Autodesk Inventor part; units mm, degrees
ref_plane "YZ Plane" through (0, 0, 0) normal (1, 0, 0) x (0, 1, 0)
ref_plane "XZ Plane" through (0, 0, 0) normal (0, 1, 0) x (-1, 0, 0)
ref_plane "XY Plane" through (0, 0, 0) normal (0, 0, 1) x (1, 0, 0)
sketch "Sketch1" plane through (0, 0, 0) normal (1, 0, 0) x (0, 1, 0)
  line L0 (0, 0) -> (47.0027, 0)
  line L1 (47.0027, 0) -> (47.0027, -9.525)
  line L2 (47.0027, -9.525) -> (0, -9.525)
  line L3 (0, -9.525) -> (0, 0)
  dimension "d0" = 47.0027
  dimension "d1" = 9.525
revolve "Revolution1" add sketch "Sketch1" angle 360 about axis through (0, 0, -9.525) along (0, 0, 1)
sketch "Sketch2" plane through (0, 0, 0) normal (0, 0, 1) x (1, 0, 0)
  circle A0 centre (0, 0) radius 39.0906
  line L0 (0, 0) -> (27.6412, 27.6412)
  line L1 (0, 0) -> (39.0906, 0) construction
  circle A1 centre (27.6412, 27.6412) radius 3.4036
  circle A2 centre (37.7586, -10.1174) radius 3.4036
  circle A3 centre (10.1174, -37.7586) radius 3.4036
  circle A4 centre (-27.6412, -27.6412) radius 3.4036
  circle A5 centre (-37.7586, 10.1174) radius 3.4036
  circle A6 centre (-10.1174, 37.7586) radius 3.4036
  point P0 (0, 0)
  dimension "d3" = 78.1812
  dimension "d4" = 45
  dimension "d5" = 6.8072
  dimension "d8" = 360
extrude "Extrusion1" cut sketch "Sketch2" against normal blind 9.525 contours A1 L0 A0 | A0 A1 | A2 A0 | A0 A2 | L0 A1 A0 | A3 A0 | A0 A3 | A6 A0 | A0 A6 | A4 A0 | A0 A4 | A5 A0 | A0 A5
sketch "Sketch3" plane through (0, 0, 0) normal (0, 0, 1) x (1, 0, 0)
  circle A0 centre (0, 0) radius 31.1277
  line L0 (0, 0) -> (-22.0106, 22.0106)
  line L1 (0, 0) -> (31.1277, 0) construction
  circle A1 centre (-27.6412, -27.6412) radius 3.4036
  circle A2 centre (-22.0106, 22.0106) radius 5.08
  circle A3 centre (-8.0564, -30.067) radius 5.08
  circle A4 centre (30.067, 8.0564) radius 5.08
  circle A5 centre (0, 0) radius 15.875
  point P0 (0, 0)
  dimension "d12" = 62.2554
  dimension "d13" = 135
  dimension "d14" = 10.16
  dimension "d17" = 360
  dimension "d21" = 31.75
extrude "Extrusion2" cut sketch "Sketch3" against normal blind 9.525 contours A5 | A4 A0 | A0 A4 | A3 A0 | A0 A3 | A2 L0 A0 | A0 A2 | A0 L0 A2
chamfer "Chamfer1" distance 0.762 angle 45 12 edges at (-15.875, 0, 0) (0, -47.0027, 0) (0, -47.0027, -9.525) (24.987, 8.0564, 0) (24.2376, 27.6412, 0) (-13.521, 37.7586, 0) (-27.0906, 22.0106, 0) (-41.1622, 10.1174, 0) (-31.0448, -27.6412, 0) (-13.1364, -30.067, 0) (6.7138, -37.7586, 0) (34.355, -10.1174, 0)
properties part number "Motor_Adapter_Flex"
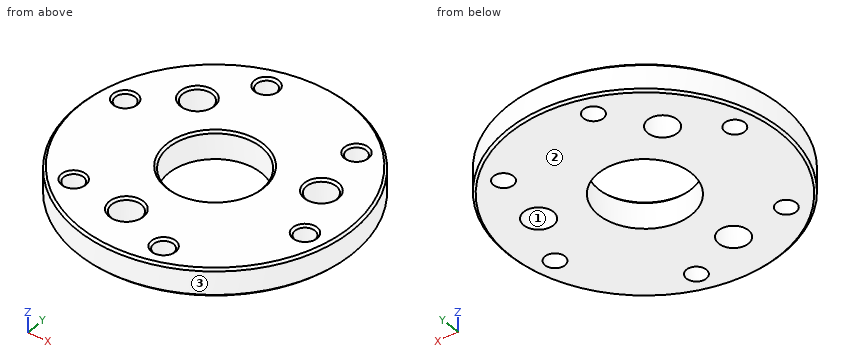
Could you check a few things on this model? Use its own coordinates, in mm. Face numbers are marked on the shaded views. Give positions to 0.01 mm unless a question says otherwise; leave off trailing zeros. Write each loop counter-clockwise with the first axis right and the second up, starting at its lowest first coordinate (ties: lowest second). Pieces come first, ordered by that corner, then holes. Notation, with made-up numbers: (37, -32) -> (81, -32) arc R29 cw to (81, -3) -> close; hole circle Ø9 at (15, 78.5). An arc over 180 degrees is marked (long way). Answer as a JSON object with one key per item and string values.
Q1. Suppose I cut it at A-A on x = 0. Write out the boundary of the cut face in (y, z) (3 decimals), then the cut area to 3 significant figures.
Taken from the geometry:
{"outline": "(-47.003, -8.763) -> (-46.241, -9.525) -> (-15.875, -9.525) -> (-15.875, -0.762) -> (-16.637, 0) -> (-46.241, 0) -> (-47.003, -0.762) -> close; (15.875, -9.525) -> (46.241, -9.525) -> (47.003, -8.763) -> (47.003, -0.762) -> (46.241, 0) -> (16.637, 0) -> (15.875, -0.762) -> close", "area": "591 mm²"}
Q2. We'd pull the mould along X, two halves only. Please class the marked faces 1, 2 and 3: released by +X, released by -X, zero draft, split by the parting line, or undercut.
Taken from the geometry:
{"face 1": "undercut", "face 2": "zero draft", "face 3": "split by the parting line"}
Q3. Please list where these lines run through material, in increasing order: L1, parallel to X at y = 0, z = -5.25 (3 decimals); L2, parallel to X at y = 26.5, z = -0.5; L3, parallel to Y at x = -3.5, z = -0.75.
Taken from the geometry:
{"L1": "x = -47.003 to -15.875, 15.875 to 47.003", "L2": "x = -38.5 to -24.91, -19.12 to 24.16, 31.12 to 38.5", "L3": "y = -46.86 to -32.34, -27.79 to -15.5, 15.5 to 46.86"}
Q4. Will these pins go through, and if not, where does the flat tip stop? pin 1 Ø3 at (x, z) = (-21, -4) entering from +Y; pin 2 Ø2 at (x, z) = (25, -8.5) entering from +Y; pin 3 Ø2 at (y, z) = (-25.5, -8) entering from -X.
Taken from the geometry:
{"pin 1": "stops at y = 42.77", "pin 2": "stops at y = 40.41", "pin 3": "stops at x = -40.11"}
